Autodesk Inventor part; units mm, degrees
ref_plane "YZ Plane" through (0, 0, 0) normal (1, 0, 0) x (0, 1, 0)
ref_plane "XZ Plane" through (0, 0, 0) normal (0, 1, 0) x (-1, 0, 0)
ref_plane "XY Plane" through (0, 0, 0) normal (0, 0, 1) x (1, 0, 0)
sketch "Skizze1" plane through (0, 0, 0) normal (0, 1, 0) x (-1, 0, 0)
  line L0 (0, 0) -> (150, 0)
  line L1 (150, 0) -> (150, -40)
  line L2 (150, -40) -> (0, -40)
  line L3 (0, -40) -> (0, 0)
  dimension "d0" = 40
  dimension "d1" = 150
extrude "Extrusion1" add sketch "Skizze1" along normal blind 3
sketch "Skizze2" plane through (0, 3, 0) normal (0, 1, 0) x (1, 0, 0)
  line L0 (-150, 0) -> (0, 0)
  line L1 (-75, 0) -> (-75, 40)
  line L2 (0, 40) -> (-150, 40)
  line L3 (-150, 40) -> (-150, 0)
  line L4 (-150, 20) -> (0, 20)
  line L5 (0, 0) -> (0, 40)
  line L6 (-13, 0) -> (-13, 40) construction
  circle A0 centre (-13, 7.5) radius 2.25
  circle A1 centre (-13, 32.5) radius 2.25
  circle A2 centre (-137, 7.5) radius 2.25
  circle A3 centre (-137, 32.5) radius 2.25
  dimension "d4" = 13
  dimension "d5" = 4.5
  dimension "d6" = 4.5
  dimension "d7" = 25
extrude "Extrusion2" cut sketch "Skizze2" against normal blind 3 contours A0 | A1 | A2 | A3
fillet "Rundung1" radius 2 4 edges at (-150, 1.5, 0) (-150, 1.5, -40) (0, 1.5, -40) (0, 1.5, 0)
properties part number "Stabilisator_05" material "PET-Kunststoff"
Source: CAD feature listing. Evaluate the final solid. Frame: model axes, mm. Give positions to 0.01 mm unless a question says otherwise; leave off trailing zeros. Loops run counter-clockwise (first coordinate to the right, second up) from the corner with the lowest first, then second, coordinate; pieces in that order, holes last. Notation, with made-up numbers: (19, -35) - (24, -35) arc R19 cw to (24, -24) - close; hole circle Ø5 at (24.5, -15.5). An arc over 180 degrees is marked (long way). Use CSV: the item, a comma, the result in double quotes. Start each with the question number.
1. Draft query along Z for faces 1 (the flat face through (-150, 1, -20)), 2 (the flat face through (-76, 1, -40)), 3 (the cylindrical face through (-134.854, 1.521, -33.176)), 4 (the flat face through (-74, 1, 0)). Return one class per face: +Z half, -Z half, draft (parallel to the pull), parting line (faces both ways), or undercut.
2. Section B-B (z = -32.5). Output: boundary loops of the cut face in (x, y), then the cut area to 3 significant figures.
3. Pin query (flat end, axial travel): pin 1 (4 mm diameter, centred on x = -137, z = -7.5, fed in from +Y). Return the tip coordinate at first contact, or that it passes through.
4. Section A-A (x = -137). Output: boundary loops of the cut face in (y, z).
5. Ray query, L1, parallel to X at y = 0.8, z = -32.5; L2, parallel to Z at x = -13, y = 2.2; L3, parallel to Z at x = -138, y = 0.95. Return the intervals inside material, ascending.
Response:
1,face 1,"draft"
1,face 2,"-Z half"
1,face 3,"undercut"
1,face 4,"+Z half"
2,outline,"(-150, 0) - (-139.25, 0) - (-139.25, 3) - (-150, 3) - close; (-134.75, 0) - (-15.25, 0) - (-15.25, 3) - (-134.75, 3) - close; (-10.75, 0) - (0, 0) - (0, 3) - (-10.75, 3) - close"
2,area,"423 mm²"
3,pin 1,"through"
4,outline,"(0, -40) - (3, -40) - (3, -34.75) - (0, -34.75) - close; (0, -30.25) - (3, -30.25) - (3, -9.75) - (0, -9.75) - close; (0, -5.25) - (3, -5.25) - (3, 0) - (0, 0) - close"
5,L1,"-150 to -139.25, -134.75 to -15.25, -10.75 to 0"
5,L2,"-40 to -34.75, -30.25 to -9.75, -5.25 to 0"
5,L3,"-40 to -34.52, -30.48 to -9.52, -5.48 to 0"
